Geometry check sheet. Reference: the model listing, model coordinates, mm. A direction names the side the tool comes from. Coordinates: 2 decimals unless noted, no trailing zeros. Write each loop counter-clockwise with the first axis right and the second up, starting at its lowest first coordinate (ties: lowest second). Pieces come first, ordered by that corner, then holes. Notation, with made-up numbers: (63.5, 6) -> (76.5, 6) arc R32 ccw to (76.5, 45) -> close; hole circle Ø8 at (69.5, 81). An arc over 180 degrees is marked (long way). Use a Markdown table: item, result.
```python
from build123d import *

# Parameters (mm, degrees)
A_BASE_T_START                                    = -1.5
A_BASE_T_OUTLINE_R                                = 47
A_BASE_T_OUTLINE_R_2                              = 1
A_BASE_T_DEPTH                                    = 3
OUTER_START                                       = -12
SKETCH2_R                                         = 50
SKETCH2_R_2                                       = 47
OUTER_RING_DEPTH                                  = 12
FINGER_BASE_THROUGH_HOLES_DEPTH                   = 72.281133549
RING_EXTRUDE_OUTLINE_R                            = 1
RING_EXTRUDE_OUTLINE_W                            = 5.516666665
RING_EXTRUDE_OUTLINE_H                            = 31.998521247
RING_EXTRUDE_OUTLINE_W_2                          = 5.516666664
RING_EXTRUDE_DEPTH                                = 3
SKETCH6_W                                         = 16.15
SKETCH6_H                                         = 4
ALLOWANCE_CUT_1_DEPTH                             = 72.281133549
ALLOWANCE_CUT_2_DEPTH                             = 6
CSK_FOR_8_FLAT_HEAD_SOCKET_CAP_SCREW1_D           = 4.9149
CSK_FOR_8_FLAT_HEAD_SOCKET_CAP_SCREW1_CSINK_D     = 9.1186
CSK_FOR_8_FLAT_HEAD_SOCKET_CAP_SCREW1_CSINK_ANGLE = 82
CLEARANCE_CONTOURING_R                            = 1


# Read off the part's stored shape, not the designer's step: a_base_t, Ring Extrude
with BuildPart() as part:
    # a_base_t outline → a_base_t (new body)
    with BuildSketch(Plane(origin=(0, 0, 0), x_dir=(1, 0, 0), z_dir=(0, 1, 0)).offset(A_BASE_T_START)):
        Circle(A_BASE_T_OUTLINE_R)
        with Locations((-17.009259258, -38.128042167)):
            Circle(A_BASE_T_OUTLINE_R_2, mode=Mode.SUBTRACT)
        with Locations((-9.166666665, -28.284271247)):
            Circle(A_BASE_T_OUTLINE_R_2, mode=Mode.SUBTRACT)
        with Locations((17.009259258, -38.128042167)):
            Circle(A_BASE_T_OUTLINE_R_2, mode=Mode.SUBTRACT)
        with Locations((27.5, -28.284271247)):
            Circle(A_BASE_T_OUTLINE_R_2, mode=Mode.SUBTRACT)
        with Locations((-27.5, 28.284271247)):
            Circle(A_BASE_T_OUTLINE_R_2, mode=Mode.SUBTRACT)
        with Locations((-17.009259258, 38.128042167)):
            Circle(A_BASE_T_OUTLINE_R_2, mode=Mode.SUBTRACT)
        with Locations((9.166666665, 28.284271247)):
            Circle(A_BASE_T_OUTLINE_R_2, mode=Mode.SUBTRACT)
        with Locations((17.009259258, 38.128042167)):
            Circle(A_BASE_T_OUTLINE_R_2, mode=Mode.SUBTRACT)
    extrude(amount=A_BASE_T_DEPTH)

    # Sketch2 → Outer Ring (add)
    with BuildSketch(Plane(origin=(0, 1.5, 0), x_dir=(1, 0, 0), z_dir=(0, 1, 0)).offset(OUTER_START)):
        with Locations(Location((0, 0, 0), (0, 0, 270))):
            Circle(SKETCH2_R)
        with Locations(Location((0, 0, 0), (0, 0, 270))):
            Circle(SKETCH2_R_2, mode=Mode.SUBTRACT)
    extrude(amount=OUTER_RING_DEPTH)

    # Sketch3 → Finger Base Through Holes (cut, through all)
    with BuildSketch(Plane.XZ.offset(1.5)):
        Polygon((35.574999997, 23.78575), (40.074999997, 23.78575), (40.074999997, 5.78575), (14.924999997, 5.78575), (14.924999997, 23.78575), (19.424999997, 23.78575), (19.424999997, 29.784271247), (35.574999997, 29.784271247), align=None)
        Polygon((-1.091666667, 29.784271247), (-17.241666667, 29.784271247), (-17.241666667, 23.78575), (-21.741666667, 23.78575), (-21.741666667, 5.78575), (3.408333333, 5.78575), (3.408333333, 23.78575), (-1.091666667, 23.78575), align=None)
        Polygon((17.241666665, -29.784271247), (1.091666665, -29.784271247), (1.091666665, -23.78575), (-3.408333335, -23.78575), (-3.408333335, -5.78575), (21.741666665, -5.78575), (21.741666665, -23.78575), (17.241666665, -23.78575), align=None)
        Polygon((-19.425, -29.784271247), (-35.575, -29.784271247), (-35.575, -23.78575), (-40.075, -23.78575), (-40.075, -5.78575), (-14.925, -5.78575), (-14.925, -23.78575), (-19.425, -23.78575), align=None)
    extrude(amount=-FINGER_BASE_THROUGH_HOLES_DEPTH, mode=Mode.SUBTRACT)

    # Ring Extrude outline → Ring Extrude (add)
    with BuildSketch(Plane.XZ.offset(1.5)):
        with BuildLine():
            Line((35.574999997, 30.715132674), (35.574999997, 23.78575))
            Line((35.574999997, 23.78575), (40.074999997, 23.78575))
            Line((40.074999997, 23.78575), (40.074999997, 1.78575))
            Line((40.074999997, 1.78575), (14.924999997, 1.78575))
            Line((14.924999997, 1.78575), (14.924999997, 23.78575))
            Line((14.924999997, 23.78575), (19.424999997, 23.78575))
            Line((19.424999997, 23.78575), (19.424999997, 33.784271247))
            Line((19.424999997, 33.784271247), (32.67450101, 33.784271247))
            ThreePointArc((32.67450101, 33.784271247), (0, 47), (-32.67450101, 33.784271247))
            Line((-32.67450101, 33.784271247), (-24.741666667, 33.784271247))
            Line((-24.741666667, 33.784271247), (-24.741666667, 1.78575))
            Line((-24.741666667, 1.78575), (-46.966063247, 1.78575))
            ThreePointArc((-46.966063247, 1.78575), (-44.354634753, -15.545622403), (-35.575, -30.715132671))
            Line((-35.575, -30.715132671), (-35.575, -23.78575))
            Line((-35.575, -23.78575), (-40.075, -23.78575))
            Line((-40.075, -23.78575), (-40.075, -1.78575))
            Line((-40.075, -1.78575), (-14.925, -1.78575))
            Line((-14.925, -1.78575), (-14.925, -23.78575))
            Line((-14.925, -23.78575), (-19.425, -23.78575))
            Line((-19.425, -23.78575), (-19.425, -33.784271247))
            Line((-19.425, -33.784271247), (-32.67450101, -33.784271247))
            ThreePointArc((-32.67450101, -33.784271247), (0, -47), (32.67450101, -33.784271247))
            Line((32.67450101, -33.784271247), (24.741666665, -33.784271247))
            Line((24.741666665, -33.784271247), (24.741666665, -1.78575))
            Line((24.741666665, -1.78575), (46.966063247, -1.78575))
            ThreePointArc((46.966063247, -1.78575), (44.354634753, 15.545622405), (35.574999997, 30.715132674))
        make_face()
        with Locations((-17.009259258, -38.128042167)):
            Circle(RING_EXTRUDE_OUTLINE_R, mode=Mode.SUBTRACT)
        with Locations((-9.166666667, -17.785010623)):
            Rectangle(RING_EXTRUDE_OUTLINE_W, RING_EXTRUDE_OUTLINE_H, mode=Mode.SUBTRACT)
        with Locations((17.009259258, -38.128042167)):
            Circle(RING_EXTRUDE_OUTLINE_R, mode=Mode.SUBTRACT)
        Polygon((17.241666665, -23.78575), (17.241666665, -33.784271247), (1.091666665, -33.784271247), (1.091666665, -23.78575), (-3.408333335, -23.78575), (-3.408333335, -1.78575), (21.741666665, -1.78575), (21.741666665, -23.78575), align=None, mode=Mode.SUBTRACT)
        Polygon((-1.091666667, 23.78575), (3.408333333, 23.78575), (3.408333333, 1.78575), (-21.741666667, 1.78575), (-21.741666667, 23.78575), (-17.241666667, 23.78575), (-17.241666667, 33.784271247), (-1.091666667, 33.784271247), align=None, mode=Mode.SUBTRACT)
        with Locations((-17.009259258, 38.128042167)):
            Circle(RING_EXTRUDE_OUTLINE_R, mode=Mode.SUBTRACT)
        with Locations((9.166666665, 17.785010623)):
            Rectangle(RING_EXTRUDE_OUTLINE_W_2, RING_EXTRUDE_OUTLINE_H, mode=Mode.SUBTRACT)
        with Locations((17.009259258, 38.128042167)):
            Circle(RING_EXTRUDE_OUTLINE_R, mode=Mode.SUBTRACT)
    extrude(amount=RING_EXTRUDE_DEPTH)

    # Sketch6 → Allowance Cut 1 (cut, through all)
    with BuildSketch(Plane.XZ.offset(1.5)):
        with Locations((27.499999997, 31.784271247)):
            Rectangle(SKETCH6_W, SKETCH6_H)
        with Locations((-27.5, -31.784271247)):
            Rectangle(SKETCH6_W, SKETCH6_H)
    extrude(amount=ALLOWANCE_CUT_1_DEPTH, mode=Mode.SUBTRACT)

    # Sketch7 → Allowance Cut 2 (cut)
    with BuildSketch(Plane.XZ.offset(10.5)):
        with BuildLine():
            Line((-38.500146082, -26.958092508), (-40.957602214, -28.678821818))
            ThreePointArc((-40.957602214, -28.678821818), (-35.355339059, -35.355339059), (-28.678821818, -40.957602214))
            Line((-28.678821818, -40.957602214), (-26.958092508, -38.500146082))
            ThreePointArc((-26.958092508, -38.500146082), (-29.909386843, -36.25504901), (-32.67450101, -33.784271247))
            Line((-32.67450101, -33.784271247), (-35.575, -33.784271247))
            Line((-35.575, -33.784271247), (-35.575, -30.715132671))
            ThreePointArc((-35.575, -30.715132671), (-37.085181063, -28.873679114), (-38.500146082, -26.958092508))
        make_face()
        with BuildLine():
            ThreePointArc((40.957602214, 28.678821818), (35.355339059, 35.355339059), (28.678821818, 40.957602214))
            Line((28.678821818, 40.957602214), (26.958092508, 38.500146082))
            ThreePointArc((26.958092508, 38.500146082), (29.909386843, 36.25504901), (32.67450101, 33.784271247))
            Line((32.67450101, 33.784271247), (35.574999997, 33.784271247))
            Line((35.574999997, 33.784271247), (35.574999997, 30.715132674))
            ThreePointArc((35.574999997, 30.715132674), (37.085181061, 28.873679115), (38.500146082, 26.958092508))
            Line((38.500146082, 26.958092508), (40.957602214, 28.678821818))
        make_face()
    extrude(amount=-ALLOWANCE_CUT_2_DEPTH, mode=Mode.SUBTRACT)

    # CSK for #8 Flat Head Socket Cap Screw1 (through all)
    with Locations(Plane(origin=(0, 1.5, 0), x_dir=(1, 0, 0), z_dir=(0, 1, 0))):
        with Locations((-17.009259258, -38.128042167), (17.009259258, -38.128042167), (17.009259258, 38.128042167), (-17.009259258, 38.128042167)):
            CounterSinkHole(CSK_FOR_8_FLAT_HEAD_SOCKET_CAP_SCREW1_D / 2, CSK_FOR_8_FLAT_HEAD_SOCKET_CAP_SCREW1_CSINK_D / 2, counter_sink_angle=CSK_FOR_8_FLAT_HEAD_SOCKET_CAP_SCREW1_CSINK_ANGLE)

    # Clearance Contouring
    clearance_contouring_edges = [part.edges().sort_by_distance(p)[0] for p in [
        (17.241666665, -1.5, -23.78575),
        (1.091666665, -1.5, -23.78575),
        (-19.425, -1.5, -23.78575),
        (-35.575, -1.5, -23.78575),
        (35.574999997, 0, 23.78575),
        (19.424999997, 0, 23.78575),
        (-1.091666667, 0, 23.78575),
        (-17.241666667, 0, 23.78575),
    ]]
    fillet(clearance_contouring_edges, radius=CLEARANCE_CONTOURING_R)


solid = part.part
```
Item 1: Tool access check on faces 3 (the flat face through (28, -3, 1.786)), 4 (the cylindrical face through (-15.059, -2.734, 39.623)). Record the directions out of +Z, -Z, +X, -X, +Y, -Y that give a thin tool (end or side, any length) a straight path to the whole face; none if there is none.
Answer block:
| item | result |
|---|---|
| face 3 | -Y |
| face 4 | +Y, -Y |
Item 2: Section check B-B on z = 0. Record the boundary of the cut face in (x, y).
Answer block:
| item | result |
|---|---|
| outline | (-50, -10.5) -> (-47, -10.5) -> (-47, -4.5) -> (47, -4.5) -> (47, -10.5) -> (50, -10.5) -> (50, 1.5) -> (-50, 1.5) -> close |
Item 3: Section check A-A on y = -8.5. Record the boundary of the cut face in (x, z), then the cut area to 3 significant figures.
Answer block:
| item | result |
|---|---|
| outline | (-40.96, -28.68) -> (-38.5, -26.96) arc R47 cw to (26.96, 38.5) -> (28.68, 40.96) arc R50 ccw to start; (-28.68, -40.96) arc R50 ccw to (40.96, 28.68) -> (38.5, 26.96) arc R47 cw to (-26.96, -38.5) -> close |
| area | 813 mm^2 |
Item 4: Thickness scan on L1, parallel to X at y = -4, z = -2 (3 decimals); L2, parallel to Z at x = 14.5, y = 0; L3, parallel to X at y = -1.25, z = -16 (3 decimals). Record the ranges inside material, lowest first. Write a range as [from, to].
Answer block:
| item | result |
|---|---|
| L1 | x = [-49.96, -40.075], [-14.925, -11.925], [-6.408, -3.408], [21.742, 24.742], [46.957, 49.96] |
| L2 | z = [-47.85, -40.2], [-36.05, -29.78], [-5.79, 36.05], [40.2, 47.85] |
| L3 | x = [-47.371, -40.075], [-14.925, -3.408], [21.742, 47.371] |
Item 5: Section check D-D on y = -3. Count the separate pieces of the cut face and the enclosed holes in it, then the cut area to 3 significant figures.
Answer block:
| item | result |
|---|---|
| separate pieces | 1 |
| enclosed holes | 12 |
| area | 3,440 mm^2 |
Item 6: Depth check by flat-ended pin: P1, Ø2, axis at x = -12.5, z = 3.5, coming from the -Y side; P2, Ø1.8, axis at x = -17, y = -1.5, coming from the +Z side; P3, Ø1.5, axis at x = 31, y = 0.5, coming from the -Z side. Enter the tip coordinate at first touch or a pass-through.
Answer block:
| item | result |
|---|---|
| P1 | stops at y = -1.5 |
| P2 | stops at z = 47.34 |
| P3 | stops at z = -39.81 |
Item 7: Mould release check, pull along X, two halves, no side actions. Record for faces 1 (the flat face through (-28, -1.5, -4)), 2 (the flat face through (-27.8, -7.5, -39.7)): +X half, -X half, draft (parallel to the pull), parting line (faces both ways), or undercut.
Answer block:
| item | result |
|---|---|
| face 1 | undercut |
| face 2 | -X half |
Item 8: Section check C-C on z = 19. Record the boundary of the cut face in (x, y) (3 decimals).
Answer block:
| item | result |
|---|---|
| outline | (-46.249, -10.5) -> (-42.988, -10.5) -> (-42.988, -1.5) -> (-24.742, -1.5) -> (-24.742, -4.5) -> (-21.742, -4.5) -> (-21.742, 1.5) -> (-46.249, 1.5) -> close; (3.408, -4.5) -> (6.408, -4.5) -> (6.408, -1.5) -> (11.925, -1.5) -> (11.925, -4.5) -> (14.925, -4.5) -> (14.925, 1.5) -> (3.408, 1.5) -> close; (40.075, -4.5) -> (42.988, -4.5) -> (42.988, -10.5) -> (46.249, -10.5) -> (46.249, 1.5) -> (40.075, 1.5) -> close |
